```python
from build123d import *

# Parameters (mm, degrees)
SKETCH_1_R          = 3
EXTRUDE_1_DEPTH     = 6
SKETCH_2_R          = 1.6
CUT_EXTRUDE_1_DEPTH = 7
SKETCH_3_R          = 3
SKETCH_3_R_2        = 1.6
CUT_EXTRUDE_2_DEPTH = 4
CUT_EXTRUDE_3_DEPTH = 4
SKETCH_6_R          = 5
CUT_EXTRUDE_4_DEPTH = 0.5
CUT_EXTRUDE_6_DEPTH = 4
EXTRUDE_START       = -0.5
SKETCH_8_R          = 3
EXTRUDE_2_DEPTH     = 0.5
SKETCH_9_R          = 1.6
EXTRUDE_3_DEPTH     = 0.5
SKETCH_10_R         = 15
CUT_EXTRUDE_7_DEPTH = 44.018891199


with BuildPart() as part:
    # 草图1 → 凸台-拉伸1 (new body)
    with BuildSketch(Plane(origin=(0, 0, 0), x_dir=(1, 0, 0), z_dir=(0, 1, 0))):
        Polygon((21.550377817, 31.75), (-21.550377817, 31.75), (-28.75, 25.230657078), (-28.75, -25.230657078), (-21.550377817, -31.75), (21.550377817, -31.75), (28.75, -25.230657078), (28.75, 25.230657078), align=None)
        with Locations(Location((2.52, -26.835, 0), (0, 0, 270))):
            Circle(SKETCH_1_R, mode=Mode.SUBTRACT)
        with Locations(Location((2.52, 26.835, 0), (0, 0, 270))):
            Circle(SKETCH_1_R, mode=Mode.SUBTRACT)
    extrude(amount=EXTRUDE_1_DEPTH)

    # 草图2 → 切除-拉伸1 (cut)
    with BuildSketch(Plane(origin=(0, 6, 0), x_dir=(1, 0, 0), z_dir=(0, 1, 0))):
        with Locations(Location((10.52, 19.2, 0), (0, 0, 270))):
            Circle(SKETCH_2_R)
        with Locations(Location((10.52, -19.2, 0), (0, 0, 270))):
            Circle(SKETCH_2_R)
    extrude(amount=-CUT_EXTRUDE_1_DEPTH, mode=Mode.SUBTRACT)

    # 草图3 → 切除-拉伸2 (cut)
    # profile 1 of 2: a face of its own
    with BuildSketch(Plane(origin=(0, 6, 0), x_dir=(1, 0, 0), z_dir=(0, 1, 0))):
        with Locations(Location((10.52, 19.2, 0), (0, 0, 270))):
            Circle(SKETCH_3_R)
        with Locations(Location((10.52, 19.2, 0), (0, 0, 270))):
            Circle(SKETCH_3_R_2, mode=Mode.SUBTRACT)
    # profile 2 of 2: a face of its own
    with BuildSketch(Plane(origin=(0, 6, 0), x_dir=(1, 0, 0), z_dir=(0, 1, 0))):
        with Locations(Location((10.52, -19.2, 0), (0, 0, 270))):
            Circle(SKETCH_3_R)
        with Locations(Location((10.52, -19.2, 0), (0, 0, 270))):
            Circle(SKETCH_3_R_2, mode=Mode.SUBTRACT)
    extrude(amount=-CUT_EXTRUDE_2_DEPTH, mode=Mode.SUBTRACT)

    # 草图5 → 切除-拉伸3 (cut)
    with BuildSketch(Plane.XZ):
        Polygon((7.138802154, 26.835), (4.829401077, 30.835), (0.210598923, 30.835), (-2.098802154, 26.835), (0.210598923, 22.835), (4.829401077, 22.835), align=None)
        Polygon((7.138802154, -26.835), (4.829401077, -22.835), (0.210598923, -22.835), (-2.098802154, -26.835), (0.210598923, -30.835), (4.829401077, -30.835), align=None)
    extrude(amount=-CUT_EXTRUDE_3_DEPTH, mode=Mode.SUBTRACT)

    # 草图6 → 切除-拉伸4 (cut)
    with BuildSketch(Plane(origin=(0, 6, 0), x_dir=(1, 0, 0), z_dir=(0, 1, 0))):
        with Locations((2.52, 26.835)):
            Circle(SKETCH_6_R)
        with Locations((2.52, -26.835)):
            Circle(SKETCH_6_R)
    extrude(amount=-CUT_EXTRUDE_4_DEPTH, mode=Mode.SUBTRACT)

    # 草图7 → 切除-拉伸6 (cut)
    with BuildSketch(Plane.XZ):
        with BuildLine():
            Line((9.771398141, -28.75), (20.393940666, -28.75))
            Line((20.393940666, -28.75), (25.75, -23.900025013))
            Line((25.75, -23.900025013), (25.75, -15))
            Line((25.75, -15), (28.75, -15))
            Line((28.75, -15), (28.75, 15))
            Line((28.75, 15), (25.75, 15))
            Line((25.75, 15), (25.75, 23.900025013))
            Line((25.75, 23.900025013), (20.393940666, 28.75))
            Line((20.393940666, 28.75), (9.771398141, 28.75))
            ThreePointArc((9.771398141, 28.75), (9.957589867, 27.800534552), (10.02, 26.835))
            ThreePointArc((10.02, 26.835), (9.972506325, 25.992296328), (9.830626806, 25.160265481))
            ThreePointArc((9.830626806, 25.160265481), (14.51147597, 23.679745482), (16.52, 19.2))
            ThreePointArc((16.52, 19.2), (10.314635532, 13.203515577), (4.534058188, 19.610488278))
            ThreePointArc((4.534058188, 19.610488278), (-2.746887228, 21.495533835), (-4.731398141, 28.75))
            Line((-4.731398141, 28.75), (-20.393940666, 28.75))
            Line((-20.393940666, 28.75), (-25.75, 23.900025013))
            Line((-25.75, 23.900025013), (-25.75, 15))
            Line((-25.75, 15), (-28.75, 15))
            Line((-28.75, 15), (-28.75, -15))
            Line((-28.75, -15), (-25.75, -15))
            Line((-25.75, -15), (-25.75, -23.900025013))
            Line((-25.75, -23.900025013), (-20.393940666, -28.75))
            Line((-20.393940666, -28.75), (-4.731398141, -28.75))
            ThreePointArc((-4.731398141, -28.75), (-2.746887228, -21.495533835), (4.534058188, -19.610488278))
            ThreePointArc((4.534058188, -19.610488278), (10.314635532, -13.203515577), (16.52, -19.2))
            ThreePointArc((16.52, -19.2), (14.51147597, -23.679745482), (9.830626806, -25.160265481))
            ThreePointArc((9.830626806, -25.160265481), (9.972506325, -25.992296328), (10.02, -26.835))
            ThreePointArc((10.02, -26.835), (9.957589867, -27.800534552), (9.771398141, -28.75))
        make_face()
    extrude(amount=-CUT_EXTRUDE_6_DEPTH, mode=Mode.SUBTRACT)

    # 草图8 → 凸台-拉伸2 (add)
    with BuildSketch(Plane(origin=(0, 5.5, 0), x_dir=(1, 0, 0), z_dir=(0, 1, 0)).offset(EXTRUDE_START)):
        with Locations(Location((2.52, 26.835, 0), (0, 0, 90))):
            Circle(SKETCH_8_R)
        with Locations(Location((2.52, -26.835, 0), (0, 0, 90))):
            Circle(SKETCH_8_R)
    extrude(amount=EXTRUDE_2_DEPTH)

    # 草图9 → 凸台-拉伸3 (add)
    with BuildSketch(Plane(origin=(0, 2, 0), x_dir=(1, 0, 0), z_dir=(0, 1, 0))):
        with Locations(Location((10.52, -19.2, 0), (0, 0, 270))):
            Circle(SKETCH_9_R)
        with Locations(Location((10.52, 19.2, 0), (0, 0, 270))):
            Circle(SKETCH_9_R)
    extrude(amount=-EXTRUDE_3_DEPTH)

    # 草图10 → 切除-拉伸7 (cut, through all)
    with BuildSketch(Plane.XZ.offset(-4)):
        with Locations(Location((0, 0, 0), (0, 0, 270))):
            Circle(SKETCH_10_R)
    extrude(amount=-CUT_EXTRUDE_7_DEPTH, mode=Mode.SUBTRACT)


solid = part.part
```
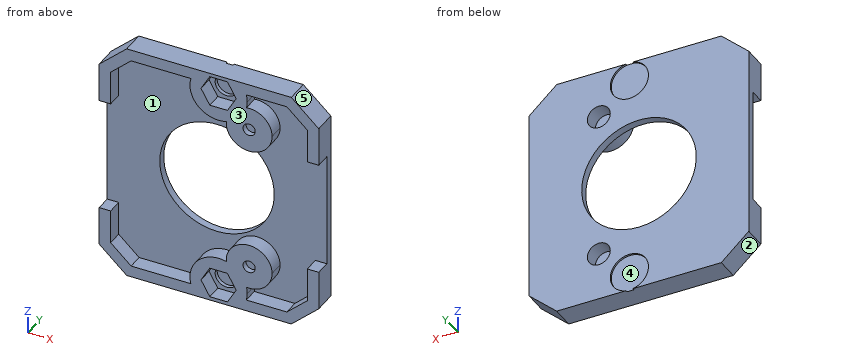
CAD build for the part. Positions are in the model's coordinates, mm. Face numbers are marked on the shaded views. A direction names the side the tool comes from. Give positions to 0.01 mm unless a question says otherwise; leave off trailing zeros. Order: outer loops, then holes, each group sorted by start corner. A loop starts at its lowest first (then second) coordinate and runs counter-clockwise, first axis right, second up.
(1) Saw through at A-A, the plane z = 0. Give the cut face in (x, y).
(2) Drill centre lines: L1, parallel to Z at x = -14, y = 1.3; L2, parallel to X at y = 0.45, z = 19.2; L3, parallel to X at y = 1.55, z = 24. Where is each one in solid material? Low to high.
(3) Mould opens along X. For the marked faces 1, 2 and 3 say: released by +X, released by -X, zero draft, split by the parting line, or undercut.
(4) Flat gauge pins, fed straight in: pin 1 (0.9 mm diameter, centred on x = 27.5, y = 2.5, fed in from +Z); pin 2 (5 mm diameter, centred on x = 10.52, z = 19.2, fed in from +Y); pin 3 (5 mm diameter, centred on x = 3, z = 29, fed in from +Y). Where does each tip first touch, or does it go through?
(5) Saw through at D-D, the plane z = 6.5. Give the cut face in (x, y), then the cut area to 3 significant figures.
(6) Saw through at B-B, the plane y = 2.8. State how many separate pieces and enclosed holes the cut face has, then the cut area to 3 significant figures.
(7) Tool access for the marked faces 4 and 5: list every direction of +Z, -Z, +X, -X, +Y, -Y with a clear straight run to the whole face (end or side of a thin tool).
Results found:
1. outline: (-28.75, 4) - (-15, 4) - (-15, 6) - (-28.75, 6) - close; (15, 4) - (28.75, 4) - (28.75, 6) - (15, 6) - close
2. L1: z = -31.75 to -28.75, 28.75 to 31.75
2. L2: x = -28.75 to -25.75, 4.52 to 8.92, 12.12 to 16.52, 25.75 to 28.75
2. L3: x = -28.75 to -25.64, -4.42 to -0.46, 5.5 to 14.12, 25.64 to 28.75
3. face 1: undercut
3. face 2: released by -X
3. face 3: zero draft
4. pin 1: stops at z = 26.77
4. pin 2: stops at y = 2
4. pin 3: stops at y = 5.5
5. outline: (-28.75, 4) - (-13.52, 4) - (-13.52, 6) - (-28.75, 6) - close; (13.52, 4) - (28.75, 4) - (28.75, 6) - (13.52, 6) - close
5. area: 60.9 mm2
6. separate pieces: 2
6. enclosed holes: 4
6. area: 735 mm2
7. face 4: +Y
7. face 5: +Z, +X, +Y, -Y
